The listing builds one solid part. Answer for the finished solid, in the listing's coordinates (mm). A direction names the side the tool comes from. Coordinates: 2 decimals unless noted, no trailing zeros. Return JSON: item names as keys, results as strings. Group by question number.
1. Which of the six approach directions +Z, -Z, +X, -X, +Y, -Y give full straight-line access (tool end or side, diameter ignored) to faces 4 (the face through (26.773, -52.256, 1.521)), 5 (the face through (33.605, -0.049, 1.521)), 6 (the face through (25.27, -86.903, 1.479)), 7 (the face through (-10.194, 37.403, 1.479)), 8 (the face through (40.824, -51.948, 1.479))?
2. The mould has two halves that part along Y. Classify faces 1 (the face through (12, 1, 0)), 2 (the face through (34.997, -75.576, 1.479)), 3 (the face through (-13, 52.1, 1.5)): pulls with the +Y half, pulls with the -Y half, needs draft (parallel to the pull), parting line crosses it, or undercut.
3. Section A-A (z = 2.4) is taken. State how many separate pieces and enclosed holes the cut face has, and give its area (3 significant figures).
4. Each of these flat-tipped pins is pushed along its axis until it touches: P1, Ø4.5, axis at x = -5.12, y = 66.81, coming from the -Z side; P2, Ø1.5, axis at y = -40, z = 1.5, coming from the -X side; P3, Ø1.5, axis at x = 9.5, z = 2.5, coming from the -Y side; P4, Ø1.5, axis at y = 51, z = 0.5, coming from the -X side. Where does it stop, or does it pass through?
5. Find the intervals of material crossed by line 1 along Y through (x, z) = (3, 2.05); line 2 along X through (y, z) = (-9, 0.2); line 3 along X through (y, z) = (54.5, 2.4), in increasing order.
```python
from build123d import *

# Parameters (mm, degrees)
SKETCH_1_R          = 4
EXTRUDE_1_DEPTH     = 3
SKETCH_3_W          = 3
SKETCH_3_H          = 10
EXTRUDE_2_DEPTH     = 3
EXTRUDE_START       = -3
EXTRUDE_3_DEPTH     = 3
SKETCH_6_W          = 3
SKETCH_6_H          = 10
EXTRUDE_4_DEPTH     = 3
SKETCH_9_R          = 2
CUT_EXTRUDE_1_DEPTH = 3
CUT_EXTRUDE_2_DEPTH = 3
SKETCH_11_R         = 2
CUT_EXTRUDE_3_DEPTH = 10
SKETCH_12_R         = 5
CUT_EXTRUDE_4_DEPTH = 10


with BuildPart() as part:
    # 草图1 → 凸台-拉伸1 (new body)
    with BuildSketch(Plane.XY):
        with BuildLine():
            Line((-14.733969043, 77.1875), (0, 0))
            ThreePointArc((0, 0), (0.234014868, -37.324654706), (-12.859683228, -72.278047703))
            ThreePointArc((-12.859683228, -72.278047703), (-12.300551756, -88.584662282), (2.8125, -94.733969043))
            ThreePointArc((2.8125, -94.733969043), (31.596681738, -75.82131672), (38.576907128, -42.094561915))
            Line((38.576907128, -42.094561915), (14.733969043, 82.8125))
            ThreePointArc((14.733969043, 82.8125), (-2.8125, 94.733969043), (-14.733969043, 77.1875))
        make_face()
        with Locations((0, 80)):
            Circle(SKETCH_1_R, mode=Mode.SUBTRACT)
        with Locations((0, -80)):
            Circle(SKETCH_1_R, mode=Mode.SUBTRACT)
    extrude(amount=EXTRUDE_1_DEPTH)

    # 草图3 → 凸台-拉伸2 (add)
    with BuildSketch(Plane(origin=(29.467938085, 5.625, 0), x_dir=(0, 0, -1), z_dir=(0.9822646028438571, 0.18749999999999992, 0))):
        with Locations((-1.5, 68.581168228)):
            Rectangle(SKETCH_3_W, SKETCH_3_H)
        with Locations((-1.5, 53.581168228)):
            Rectangle(SKETCH_3_W, SKETCH_3_H)
        with Locations((-1.5, 38.581168228)):
            Rectangle(SKETCH_3_W, SKETCH_3_H)
        with Locations((-1.5, 23.581168228)):
            Rectangle(SKETCH_3_W, SKETCH_3_H)
        with Locations((-1.5, 8.581168228)):
            Rectangle(SKETCH_3_W, SKETCH_3_H)
        with Locations((-1.5, -6.418831772)):
            Rectangle(SKETCH_3_W, SKETCH_3_H)
        with Locations((-1.5, -21.418831772)):
            Rectangle(SKETCH_3_W, SKETCH_3_H)
        with Locations((-1.5, -36.418831772)):
            Rectangle(SKETCH_3_W, SKETCH_3_H)
    extrude(amount=EXTRUDE_2_DEPTH)

    # 草图5 → 凸台-拉伸3 (add)
    with BuildSketch(Plane.XY.offset(3).offset(EXTRUDE_START)):
        with BuildLine():
            Line((41.937087865, -56.870590681), (39.020842697, -56.166663045))
            ThreePointArc((39.020842697, -56.166663045), (38.118677527, -61.090976463), (36.675111125, -65.884605639))
            Line((36.675111125, -65.884605639), (39.591356294, -66.588533275))
            Line((39.591356294, -66.588533275), (41.937087865, -56.870590681))
        make_face()
        with BuildLine():
            ThreePointArc((36.675111125, -65.884605639), (38.118677527, -61.090976463), (39.020842697, -56.166663045))
            Line((39.020842697, -56.166663045), (31.045751878, -56.518626863))
            Line((31.045751878, -56.518626863), (36.675111125, -65.884605639))
        make_face()
        with BuildLine():
            Line((35.852417991, -52.061745464), (39.348993243, -52.061745464))
            ThreePointArc((39.348993243, -52.061745464), (39.240593596, -47.056646648), (38.576907128, -42.094561915))
            Line((38.576907128, -42.094561915), (35.852417991, -52.061745464))
        make_face()
        with BuildLine():
            ThreePointArc((38.576907128, -42.094561915), (39.240593596, -47.056646648), (39.348993243, -52.061745464))
            Line((39.348993243, -52.061745464), (42.340032816, -51.830051112))
            Line((42.340032816, -51.830051112), (41.567946701, -41.862867564))
            Line((41.567946701, -41.862867564), (38.576907128, -42.094561915))
        make_face()
        with BuildLine():
            ThreePointArc((29.860599408, -78.204651867), (32.714825521, -74.091726153), (35.094532117, -69.687210158))
            Line((35.094532117, -69.687210158), (30.758010447, -62.472220292))
            Line((30.758010447, -62.472220292), (29.860599408, -78.204651867))
        make_face()
        with BuildLine():
            Line((37.650520485, -71.25785444), (35.094532117, -69.687210158))
            ThreePointArc((35.094532117, -69.687210158), (32.714825521, -74.091726153), (29.860599408, -78.204651867))
            Line((29.860599408, -78.204651867), (32.416587776, -79.775296149))
            Line((32.416587776, -79.775296149), (37.650520485, -71.25785444))
        make_face()
        with BuildLine():
            ThreePointArc((19.572509978, -87.815912184), (23.558004264, -84.786291758), (27.182310023, -81.332717899))
            Line((27.182310023, -81.332717899), (19.572509978, -65.497664614))
            Line((19.572509978, -65.497664614), (19.572509978, -87.815912184))
        make_face()
        with BuildLine():
            Line((29.127843641, -83.616333222), (27.182310023, -81.332717899))
            ThreePointArc((27.182310023, -81.332717899), (23.558004264, -84.786291758), (19.572509978, -87.815912184))
            Line((19.572509978, -87.815912184), (21.518043596, -90.099527507))
            Line((21.518043596, -90.099527507), (29.127843641, -83.616333222))
        make_face()
    extrude(amount=EXTRUDE_3_DEPTH)

    # 草图6 → 凸台-拉伸4 (add)
    with BuildSketch(Plane(origin=(0, 0, 0), x_dir=(0, 0, 1), z_dir=(-0.9822646028438571, -0.18749999999999994, 0))):
        with Locations((1.5, 68.581168228)):
            Rectangle(SKETCH_6_W, SKETCH_6_H)
        with Locations((1.5, 53.581168228)):
            Rectangle(SKETCH_6_W, SKETCH_6_H)
        with Locations((1.5, 38.581168228)):
            Rectangle(SKETCH_6_W, SKETCH_6_H)
        with Locations((1.5, 23.581168228)):
            Rectangle(SKETCH_6_W, SKETCH_6_H)
        with Locations((1.5, 8.581168228)):
            Rectangle(SKETCH_6_W, SKETCH_6_H)
    extrude(amount=EXTRUDE_4_DEPTH)

    # 草图9 → 切除-拉伸1 (cut)
    with BuildSketch(Plane.XY.offset(3)):
        with Locations((11.891030957, -62.294073604)):
            Circle(SKETCH_9_R)
        with Locations((8.750405957, -45.841141506)):
            Circle(SKETCH_9_R)
    extrude(amount=-CUT_EXTRUDE_1_DEPTH, mode=Mode.SUBTRACT)

    # 草图10 → 切除-拉伸2 (cut)
    with BuildSketch(Plane.XY.offset(3)):
        Polygon((7.5, 40.709415886), (8.973396904, 40.990665886), (10.848396904, 31.168019858), (7.901603096, 30.605519858), (6.026603096, 40.428165886), align=None)
        Polygon((10.3125, 25.975446844), (11.785896904, 26.256696844), (13.660896904, 16.434050815), (10.714103096, 15.871550815), (8.839103096, 25.694196844), align=None)
        Polygon((13.125, 11.241477801), (14.598396904, 11.522727801), (16.473396904, 1.700081772), (13.526603096, 1.137581772), (11.651603096, 10.960227801), align=None)
        Polygon((15.9375, -3.492491242), (17.410896904, -3.211241242), (19.285896904, -13.03388727), (16.339103096, -13.59638727), (14.464103096, -3.773741242), align=None)
        Polygon((18.75, -18.226460284), (20.223396904, -17.945210284), (22.098396904, -27.767856313), (19.151603096, -28.330356313), (17.410896904, -18.482075553), align=None)
        Polygon((21.5625, -32.960429327), (23.035896904, -32.679179327), (24.910896904, -42.501825355), (21.964103096, -43.064325355), (20.089103096, -33.241679327), align=None)
        Polygon((24.375, -47.69439837), (25.848396904, -47.41314837), (27.723396904, -57.235794398), (24.776603096, -57.798294398), (22.901603096, -47.97564837), align=None)
    extrude(amount=-CUT_EXTRUDE_2_DEPTH, mode=Mode.SUBTRACT)

    # 草图11 → 切除-拉伸3 (cut)
    with BuildSketch(Plane.XY.offset(3)):
        with Locations((9.616984521, 69.619074766)):
            Circle(SKETCH_11_R)
        with Locations((12.241984521, 55.867370326)):
            Circle(SKETCH_11_R)
        with Locations((-5.116984521, 66.806574766)):
            Circle(SKETCH_11_R)
        with Locations((-2.491984521, 53.054870326)):
            Circle(SKETCH_11_R)
    extrude(amount=-CUT_EXTRUDE_3_DEPTH, mode=Mode.SUBTRACT)

    # 草图12 → 切除-拉伸4 (cut)
    with BuildSketch(Plane.XY.offset(3)):
        with Locations((0, 80)):
            Circle(SKETCH_12_R)
    extrude(amount=-CUT_EXTRUDE_4_DEPTH, mode=Mode.SUBTRACT)


solid = part.part
```
The answers:
{
 "1": {"face 4": "+Z, -Z", "face 5": "+Z, -Z, +X, +Y", "face 6": "+Z, -Z, +X, -Y", "face 7": "+Z, -Z, -X", "face 8": "+Z, -Z, +X"},
 "2": {"face 1": "needs draft", "face 2": "pulls with the -Y half", "face 3": "undercut"},
 "3": {"separate pieces": "1", "enclosed holes": "15", "area": "6,430 mm2"},
 "4": {"P1": "stops at z = 0", "P2": "stops at x = -0.44", "P3": "stops at y = -93.17", "P4": "stops at x = -12.93"},
 "5": {"line 1": "y = -94.7 to -82.65, -77.35 to 76, 84 to 94.7", "line 2": "x = 1.31 to 15.46, 18.52 to 32.26", "line 3": "x = -13.46 to -3.87, -1.11 to 10.78, 13.7 to 23.19"}
}
